```python
from build123d import *

# Parameters (mm, degrees)
SKETCH_W        = 50
SKETCH_H        = 50
PAD_DEPTH       = 50
SKETCH001_R     = 19
POCKET_DEPTH    = 45
SKETCH002_W     = 50
SKETCH002_H     = 25
POCKET001_DEPTH = 45
SKETCH003_R     = 10.5
SKETCH003_R_2   = 1.5
POCKET002_DEPTH = 5.001
SKETCH004_W     = 6
SKETCH004_H     = 45
PAD001_DEPTH    = 25
SKETCH005_R     = 5
POCKET003_DEPTH = 12
SKETCH006_R     = 2.55
POCKET004_DEPTH = 3.001


with BuildPart() as part:
    # Sketch → Pad (new body)
    with BuildSketch(Plane.XY):
        Rectangle(SKETCH_W, SKETCH_H)
    extrude(amount=PAD_DEPTH)

    # Sketch001 (on DatumPlane) → Pocket (cut)
    with BuildSketch(Plane.XY.offset(50)):
        Circle(SKETCH001_R)
    extrude(amount=-POCKET_DEPTH, mode=Mode.SUBTRACT)

    # Sketch002 (on DatumPlane) → Pocket001 (cut)
    with BuildSketch(Plane.XY.offset(50)):
        with Locations((0, 12.5)):
            Rectangle(SKETCH002_W, SKETCH002_H)
    extrude(amount=-POCKET001_DEPTH, mode=Mode.SUBTRACT)

    # Sketch003 (on DatumPlane) → Pocket002 (cut, through all)
    with BuildSketch(Plane.XY.offset(5)):
        Circle(SKETCH003_R)
        with Locations((0, -15)):
            Circle(SKETCH003_R_2)
        with Locations((12.990381, 7.5)):
            Circle(SKETCH003_R_2)
        with Locations((-12.99, 7.5)):
            Circle(SKETCH003_R_2)
    extrude(amount=-POCKET002_DEPTH, mode=Mode.SUBTRACT)

    # Sketch004 (on DatumPlane) → Pad001 (join)
    with BuildSketch(Plane(origin=(0, 0, 0), x_dir=(-1, 0, 0), z_dir=(0, 1, 0))):
        with Locations((-22, 27.5)):
            Rectangle(SKETCH004_W, SKETCH004_H)
        with Locations((22, 27.5)):
            Rectangle(SKETCH004_W, SKETCH004_H)
    extrude(amount=PAD001_DEPTH)

    # Sketch005 (on DatumPlane) → Pocket003 (cut)
    with BuildSketch(Plane(origin=(0, -10, 0), x_dir=(-1, 0, 0), z_dir=(0, 1, 0))):
        with Locations((0, 35)):
            Circle(SKETCH005_R)
        with Locations((0, 15)):
            Circle(SKETCH005_R)
        with Locations((10, 25)):
            Circle(SKETCH005_R)
        with Locations((-10, 25)):
            Circle(SKETCH005_R)
    extrude(amount=-POCKET003_DEPTH, mode=Mode.SUBTRACT)

    # Sketch006 (on DatumPlane) → Pocket004 (cut, through all)
    with BuildSketch(Plane(origin=(0, -22, 0), x_dir=(-1, 0, 0), z_dir=(0, 1, 0))):
        with Locations((0, 15)):
            Circle(SKETCH006_R)
        with Locations((10, 25)):
            Circle(SKETCH006_R)
        with Locations((0, 35)):
            Circle(SKETCH006_R)
        with Locations((-10, 25)):
            Circle(SKETCH006_R)
    extrude(amount=-POCKET004_DEPTH, mode=Mode.SUBTRACT)


solid = part.part
```
CAD build for the part. Positions are in the model's coordinates, mm. A direction names the side the tool comes from. Round coordinates to 2 decimals unless told otherwise and drop trailing zeros. Order: outer loops, then holes, each group sorted by start corner. A loop starts at its lowest first (then second) coordinate and runs counter-clockwise, first axis right, second up. Notation, with made-up numbers: (68.25, -23.5) - (114.25, -23.5) arc R18 ccw to (114.25, -1.5) - close; hole circle Ø7 at (53, 88.5). An arc over 180 degrees is marked (long way). Answer as CSV lines item,"result". Start each with the question number.
1. Saw through at B-B, the plane z = 15. Write the cut outline in (x, y).
2. Saw through at D-D, the plane y = 7.5. Write the cut outline in (x, z).
3. Tool access for faces 5 (the face through (19, 12, 27)), 6 (the face through (-4.619, -20.139, 13.085)), 7 (the face through (14.38, 6.93, 2.54)): list every direction of +Z, -Z, +X, -X, +Y, -Y with a clear straight run to the whole face (end or side of a thin tool).
4. Drill centre lines: L1, parallel to Z at x = 0, y = -22.8; L2, parallel to Z at x = 0, y = -20.2; L3, parallel to X at y = 7, z = 3. Where is each one in solid material? Low to high. Write a range as [from, to].
5. Saw through at C-C, the plane y = -1. Write the cut outline in (x, z), and give its area (3 significant figures).
6. Pull direction Y, two halves, no side cores. Call faces 1 (the face through (-2, -22, 33)), 2 (the face through (-0.325, -16.464, 2.535)), 3 (the face through (-25, 0, 25)), 4 (the face through (0, -25, 25)): +Y half, -Y half, draft (parallel to the pull), parting line (faces both ways), or undercut.
7. Saw through at A-A, the plane x = 0. Count the separate pieces of the cut face and the enclosed holes in it, and give its area (3 significant figures).
8. Pin check, flat tips, straight feed: pin 1 (19 mm diameter, centred on x = -2.5, y = 1, fed in from +Z); pin 2 (5 mm diameter, centred on x = -0.5, z = 36.5, fed in from +Y). Stop position of each tip, or through.
Model answer:
1,outline,"(-25, -25) - (-2.55, -25) - (-2.55, -22) - (-5, -22) - (-5, -18.33) arc R19 cw to (-19, 0) - (-19, 25) - (-25, 25) - close; (2.55, -25) - (25, -25) - (25, 25) - (19, 25) - (19, 0) arc R19 cw to (5, -18.33) - (5, -22) - (2.55, -22) - close"
2,outline,"(-25, 0) - (-14.49, 0) - (-14.49, 5) - (-19, 5) - (-19, 50) - (-25, 50) - close; (-11.49, 0) - (-7.35, 0) - (-7.35, 5) - (-11.49, 5) - close; (7.35, 0) - (11.49, 0) - (11.49, 5) - (7.35, 5) - close; (14.49, 0) - (25, 0) - (25, 50) - (19, 50) - (19, 5) - (14.49, 5) - close"
3,face 5,"+Z, +Y"
3,face 6,"+Y"
3,face 7,"+Z, -Z"
4,L1,"z = [0, 12.45], [17.55, 32.45], [37.55, 50]"
4,L2,"z = [0, 10], [20, 30], [40, 50]"
4,L3,"x = [-25, -14.4], [-11.58, -7.83], [7.83, 11.58], [14.4, 25]"
5,outline,"(-25, 0) - (-10.45, 0) - (-10.45, 5) - (-18.97, 5) - (-18.97, 50) - (-25, 50) - close; (10.45, 0) - (25, 0) - (25, 50) - (18.97, 50) - (18.97, 5) - (10.45, 5) - close"
5,area,"688 mm²"
6,face 1,"+Y half"
6,face 2,"undercut"
6,face 3,"draft"
6,face 4,"-Y half"
7,separate pieces,"5"
7,enclosed holes,"0"
7,area,"309 mm²"
8,pin 1,"stops at z = 5"
8,pin 2,"stops at y = -22"
